```python
from build123d import *

# Parameters (mm, degrees)
SKETCH_2_R          = 2.5
EXTRUDE_1_DEPTH     = 8
CUT_EXTRUDE_START   = -5.8
CUT_EXTRUDE_1_DEPTH = 5.8


with BuildPart() as part:
    # 草图2 → 凸台-拉伸1 (new body)
    with BuildSketch(Plane(origin=(0, 0, 4.385209583), x_dir=(-1, 0, 0), z_dir=(0, 0, -1))):
        with Locations((-50.023496645, 46.50258845)):
            Circle(SKETCH_2_R)
    extrude(amount=EXTRUDE_1_DEPTH)

    # 草图3 → 切除-拉伸1 (cut)
    with BuildSketch(Plane(origin=(0, 0, -3.614790417), x_dir=(-1, 0, 0), z_dir=(0, 0, -1)).offset(CUT_EXTRUDE_START)):
        with BuildLine():
            Line((-51.564528211, 48.471146733), (-51.564528211, 44.534030167))
            ThreePointArc((-51.564528211, 44.534030167), (-52.523496645, 46.50258845), (-51.564528211, 48.471146733))
        make_face()
        with BuildLine():
            Line((-48.564528211, 48.532714335), (-48.564528211, 44.472462565))
            ThreePointArc((-48.564528211, 44.472462565), (-47.523496645, 46.50258845), (-48.564528211, 48.532714335))
        make_face()
    extrude(amount=CUT_EXTRUDE_1_DEPTH, mode=Mode.SUBTRACT)


solid = part.part
```
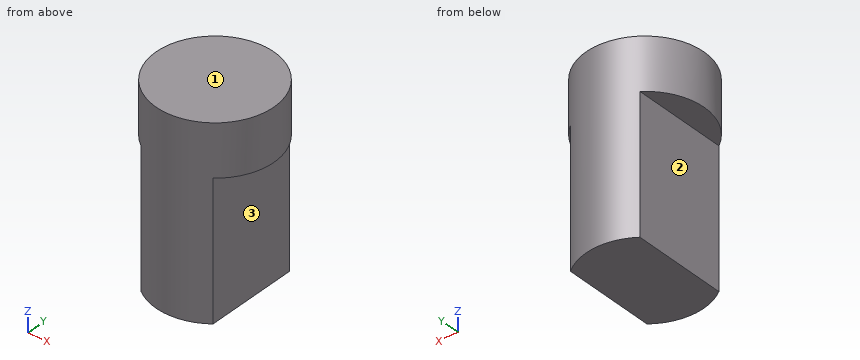
For this review, take the finished solid that the model builds, in its own axes (mm). Face numbers are marked on the shaded views. A direction names the side the tool comes from. Give positions to 0.01 mm unless a question says otherwise; leave off trailing zeros. Write each loop counter-clockwise with the first axis right and the second up, starting at its lowest first coordinate (ties: lowest second). Pieces come first, ordered by that corner, then holes. Notation, with made-up numbers: M -26.5,27.5 L 9.5,27.5 A29 cw 9.5,65.5 Z; hole C 28,66 d9. An arc over 180 degrees is marked long. Answer as a JSON object with one key per item and string values. Group by question number.
Item 1: Tool access review of the marked faces 1, 2 and 3: name each direction out of +Z, -Z, +X, -X, +Y, -Y from which nothing blocks a thin tool from reaching the whole face with its end or side.
Item 2: Consider section A-A on y = 47.8. Write out the cut boundary in (x, z).
Item 3: For probe 1 along X at (y, z) = (47.25, 0.5); probe 2 along Z at (x, y) = (48.4, 47.5); probe 3 along Y at (x, z) = (50.85, -1.5), list the stretches that pass through material, from the lowest coordinate up. Write a range as [from, to].
Item 4: Consider section D-D on y = 45.85. Write out the cut boundary in (x, z), plus the area to 3 significant figures.
Item 5: Consider section C-C on x = 51.65. Write out the cut boundary in (y, z), plus the area to 3 significant figures.
Item 6: For pin 1 Ø1 at (y, z) = (45, -1.5) entering from +X; pin 2 Ø2 at (x, z) = (51.5, -2) entering from +Y; pin 3 Ø0.5 at (x, y) = (52, 46) entering from -Z, all flat-tipped, find the tip position at first contact; note any pin that passes through.
Item 7: Consider section B-B on z = 1.5. Write out the cut boundary in (x, y).
Check result:
{
 "1": {"face 1": "+Z, +X, -X, +Y, -Y", "face 2": "-Z, -X, +Y, -Y", "face 3": "-Z, +X, +Y, -Y"},
 "2": {"outline": "M 47.89,2.19 L 48.56,2.19 L 48.56,-3.61 L 51.56,-3.61 L 51.56,2.19 L 52.16,2.19 L 52.16,4.39 L 47.89,4.39 Z"},
 "3": {"probe 1": "x = [48.56, 51.56]", "probe 2": "z = [2.19, 4.39]", "probe 3": "y = [44.14, 48.86]"},
 "4": {"outline": "M 47.61,2.19 L 48.56,2.19 L 48.56,-3.61 L 51.56,-3.61 L 51.56,2.19 L 52.44,2.19 L 52.44,4.39 L 47.61,4.39 Z", "area": "28.0 mm^2"},
 "5": {"outline": "M 44.6,2.19 L 48.4,2.19 L 48.4,4.39 L 44.6,4.39 Z", "area": "8.35 mm^2"},
 "6": {"pin 1": "stops at x = 51.56", "pin 2": "stops at y = 48.96", "pin 3": "stops at z = 2.19"},
 "7": {"outline": "M 48.56,44.47 A2.5 ccw 51.56,44.53 L 51.56,48.47 A2.5 ccw 48.56,48.53 Z"}
}
